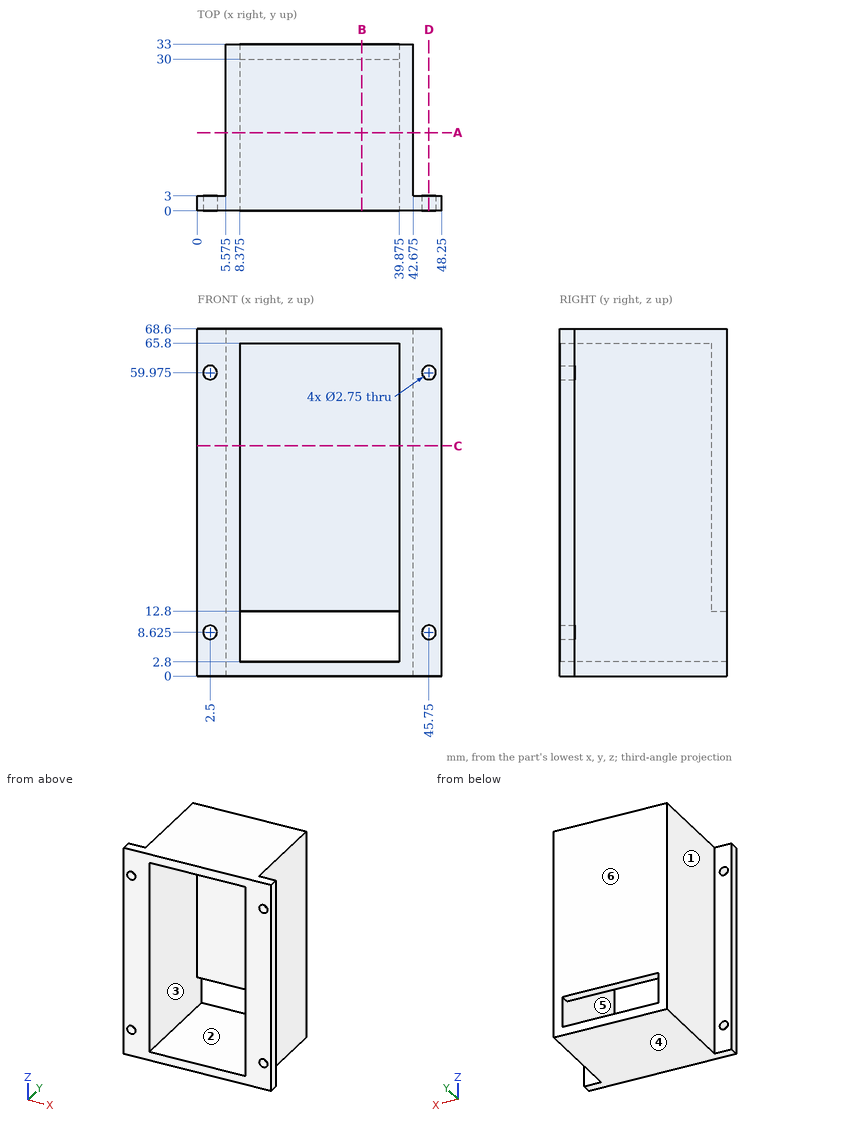
Can you work these out from the drawing? Everything is in mm from the part's minimum corner. A direction names the side the tool comes from. Round coordinates to 2 decimals unless told otherwise and drop trailing zeros. Order: outer loops, then holes, each group sorted by start corner. A loop starts at its lowest first (then second) coordinate and runs counter-clockwise, first axis right, second up. Notation, with made-up numbers: (3.25, 9.5) -> (60.25, 9.5) arc R23 ccw to (60.25, 40.5) -> close; hole circle Ø6 at (53, -27). An arc over 180 degrees is marked (long way). Return JSON: item names as keys, results as strings. Group by question number.
1. We'd pull the mould along Z, two halves only. Please class the marked faces 4, 5 and 6: released by +Z, released by -Z, zero draft, split by the parting line, or undercut.
2. If we section it at A-A, the plane y = 15.5: Write out the boundary of the cut face in (x, z) (3 decimals).
3. If we section it at D-D, the plane x = 45.75: Write out the boundary of the cut face in (y, z), then the cut area to 3 significant figures.
4. If we section it at B-B, the plane x = 32.5: Write out the boundary of the cut face in (y, z), then the cut area to 3 significant figures.
5. If we section it at C-C, the plane z = 45.5: Write out the boundary of the cut face in (x, y) (3 decimals).
6. I need wall thicknesses on line 1 (Z direction, x = 28, y = 12); line 2 (X direction, y = 25.5, z = 43) (3 decimals); line 3 (Z direction, x = 11.5, y = 31). Which ranges of each line are inside material? Lowest first, please. Write a range as [from, to].
7. Which directions (+Z, -Z, +X, -X, +Y, -Y) give clear straight access to the entire face, cutting with the end or side of a thin tool? Please do the marked faces 1, 2 and 3.
8. Will these pins go through, and if not, where does the flat tip stop? pin 1 (4.5 mm diameter, centred on x = 45.75, z = 8.625, fed in from +Y); pin 2 (2 mm diameter, centred on y = 18.5, z = 58.5, fed in from +X) (3 decimals); pin 3 (5 mm diameter, centred on x = 16, y = 14, fed in from -Z); pin 4 (10 mm diameter, centred on y = 22, z = 49, fed in from -X) (3 decimals).
Output values:
{
 "1": {"face 4": "released by -Z", "face 5": "undercut", "face 6": "zero draft"},
 "2": {"outline": "(5.575, 0) -> (42.675, 0) -> (42.675, 68.6) -> (5.575, 68.6) -> close; hole (8.375, 2.8) -> (39.875, 2.8) -> (39.875, 65.8) -> (8.375, 65.8) -> close"},
 "3": {"outline": "(0, 0) -> (3, 0) -> (3, 7.25) -> (0, 7.25) -> close; (0, 10) -> (3, 10) -> (3, 58.6) -> (0, 58.6) -> close; (0, 61.35) -> (3, 61.35) -> (3, 68.6) -> (0, 68.6) -> close", "area": "189 mm²"},
 "4": {"outline": "(0, 0) -> (33, 0) -> (33, 2.8) -> (0, 2.8) -> close; (0, 65.8) -> (30, 65.8) -> (30, 12.8) -> (33, 12.8) -> (33, 68.6) -> (0, 68.6) -> close", "area": "344 mm²"},
 "5": {"outline": "(0, 0) -> (8.375, 0) -> (8.375, 30) -> (39.875, 30) -> (39.875, 0) -> (48.25, 0) -> (48.25, 3) -> (42.675, 3) -> (42.675, 33) -> (5.575, 33) -> (5.575, 3) -> (0, 3) -> close"},
 "6": {"line 1": "[0, 2.8], [65.8, 68.6]", "line 2": "[5.575, 8.375], [39.875, 42.675]", "line 3": "[0, 2.8], [12.8, 68.6]"},
 "7": {"face 1": "+Z, -Z, -X, +Y", "face 2": "+Y, -Y", "face 3": "-Y"},
 "8": {"pin 1": "y = 3", "pin 2": "x = 42.675", "pin 3": "z = 0", "pin 4": "x = 5.575"}
}
